Drawing for the job (mm, zero at the part's lowest x, y, z). Round coordinates to 2 decimals unless told otherwise and drop trailing zeros. Write each loop counter-clockwise with the first axis right and the second up, starting at its lowest first coordinate (ties: lowest second). Pieces come first, ordered by that corner, then holes.
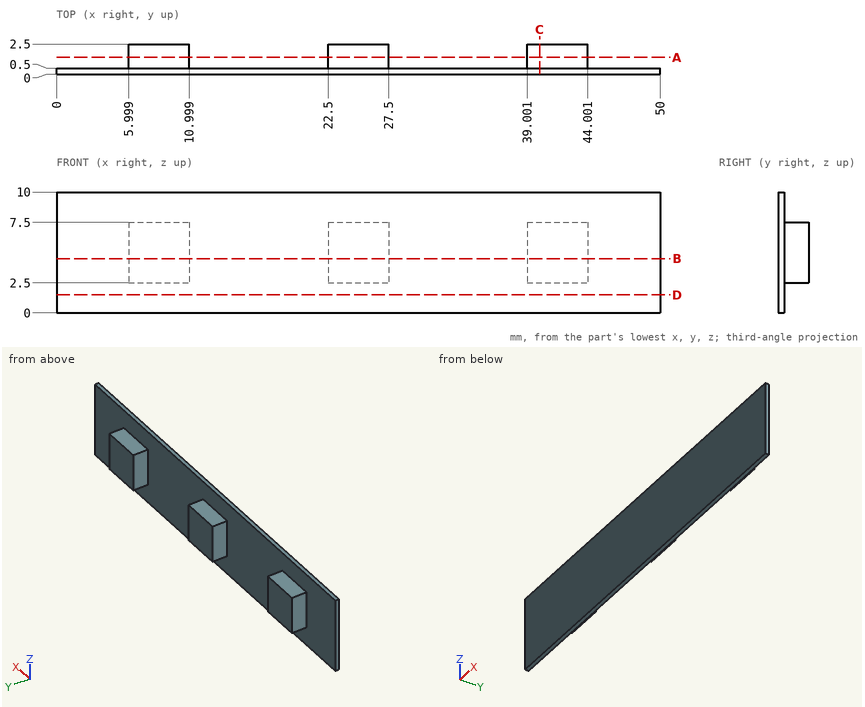
1) Cut at C-C on x = 40. List the corners of the cut face in (y, z).
2) Cut at B-B on z = 4.5. List the corners of the cut face in (x, y).
3) Flat gauge pins, fed straight in: pin 1 Ø0.6 at (y, z) = (1.5, 6) entering from -X; pin 2 Ø0.6 at (x, y) = (41.5, 1) entering from +Z. Where does each tip first touch, or does it go through?
4) Wall check: probe 1 along X at (y, z) = (2.35, 4); probe 2 along Z at (x, y) = (41, 1.55); probe 3 along Y at (x, z) = (18, 5.25). Give the ranges that are in metal, low to high.
5) Cut at D-D on z = 1.5. List the corners of the cut face in (x, y).
6) Cut at A-A on y = 1.4. List the corners of the cut face in (x, z), and give its area (3 significant figures).
Result sheet:
1. outline: (0, 0) - (0.5, 0) - (0.5, 2.5) - (2.5, 2.5) - (2.5, 7.5) - (0.5, 7.5) - (0.5, 10) - (0, 10) - close
2. outline: (0, 0) - (50, 0) - (50, 0.5) - (44, 0.5) - (44, 2.5) - (39, 2.5) - (39, 0.5) - (27.5, 0.5) - (27.5, 2.5) - (22.5, 2.5) - (22.5, 0.5) - (11, 0.5) - (11, 2.5) - (6, 2.5) - (6, 0.5) - (0, 0.5) - close
3. pin 1: stops at x = 6
3. pin 2: stops at z = 7.5
4. probe 1: x = 6 to 11, 22.5 to 27.5, 39 to 44
4. probe 2: z = 2.5 to 7.5
4. probe 3: y = 0 to 0.5
5. outline: (0, 0) - (50, 0) - (50, 0.5) - (0, 0.5) - close
6. outline: (6, 2.5) - (11, 2.5) - (11, 7.5) - (6, 7.5) - close; (22.5, 2.5) - (27.5, 2.5) - (27.5, 7.5) - (22.5, 7.5) - close; (39, 2.5) - (44, 2.5) - (44, 7.5) - (39, 7.5) - close
6. area: 75.0 mm2
